```python
from build123d import *

# Parameters (mm, degrees)
SKETCH1_R           = 13.1
BOSS_EXTRUDE1_DEPTH = 47.8
SKETCH2_R           = 10
BOSS_EXTRUDE2_DEPTH = 0.4
SKETCH3_R           = 4
BOSS_EXTRUDE3_DEPTH = 1.4
CHAMFER2_SIZE       = 1.4
CHAMFER3_SIZE       = 0.4
SKETCH4_R           = 9
BOSS_EXTRUDE4_DEPTH = 0.4
CHAMFER4_SIZE       = 0.4
WRAP1_START         = 40.976923077
WRAP1_DEPTH         = 4.31474359
WRAP1_START_2       = 42.849358974
WRAP1_2_DEPTH       = 0.569871795
WRAP1_START_3       = 2.116666667
WRAP1_3_DEPTH       = 0.651282051


# Read off the part's stored shape, not the designer's step: Wrap1
with BuildPart() as part:
    # Sketch1 → Boss-Extrude1 (new body)
    with BuildSketch(Plane(origin=(0, 0, 0), x_dir=(1, 0, 0), z_dir=(0, 1, 0))):
        with Locations(Location((0, 0, 0), (0, 0, 90))):
            Circle(SKETCH1_R)
    extrude(amount=BOSS_EXTRUDE1_DEPTH)

    # Sketch2 → Boss-Extrude2 (add)
    with BuildSketch(Plane(origin=(0, 47.8, 0), x_dir=(1, 0, 0), z_dir=(0, 1, 0))):
        with Locations(Location((0, 0, 0), (0, 0, 270))):
            Circle(SKETCH2_R)
    extrude(amount=BOSS_EXTRUDE2_DEPTH)

    # Sketch3 → Boss-Extrude3 (add)
    with BuildSketch(Plane(origin=(0, 48.2, 0), x_dir=(1, 0, 0), z_dir=(0, 1, 0))):
        with Locations(Location((0, 0, 0), (0, 0, 270))):
            Circle(SKETCH3_R)
    extrude(amount=BOSS_EXTRUDE3_DEPTH)

    # Chamfer2
    chamfer2_edges = [part.edges().sort_by_distance(p)[0] for p in [
        (0, 48.2, -4),
    ]]
    chamfer(chamfer2_edges, length=CHAMFER2_SIZE - 0.0001)  # a hair under: the kernel refuses the full size

    # Chamfer3
    chamfer3_edges = [part.edges().sort_by_distance(p)[0] for p in [
        (0, 47.8, -10),
    ]]
    chamfer(chamfer3_edges, length=CHAMFER3_SIZE - 0.0001)  # a hair under: the kernel refuses the full size

    # Sketch4 → Boss-Extrude4 (add)
    with BuildSketch(Plane.XZ):
        with Locations(Location((0, 0, 0), (0, 0, 90))):
            Circle(SKETCH4_R)
    extrude(amount=BOSS_EXTRUDE4_DEPTH)

    # Chamfer4
    chamfer4_edges = [part.edges().sort_by_distance(p)[0] for p in [
        (0, 0, -9),
    ]]
    chamfer(chamfer4_edges, length=CHAMFER4_SIZE - 0.0001)  # a hair under: the kernel refuses the full size

    # Wrap1 outline → Wrap1 (add)
    with BuildSketch(Plane(origin=(0, 0, 0), x_dir=(1, 0, 0), z_dir=(0, 1, 0)).offset(WRAP1_START)):
        with BuildLine():
            Line((2.348137979, -12.887833333), (2.34993045, -12.897671375))
            ThreePointArc((2.34993045, -12.897671375), (2.62988756, -12.843511647), (2.908600522, -12.783275911))
            Line((2.908600522, -12.783275911), (2.906381909, -12.773525128))
            ThreePointArc((2.906381909, -12.773525128), (2.627881543, -12.833714918), (2.348137979, -12.887833333))
        make_face()
    extrude(amount=WRAP1_DEPTH)

    # Wrap1 2 outline → Wrap1 2 (add)
    with BuildSketch(Plane(origin=(0, 0, 0), x_dir=(1, 0, 0), z_dir=(0, 1, 0)).offset(WRAP1_START_2)):
        with BuildLine():
            ThreePointArc((0.488721144, -13.100887437), (1.422958155, -13.032547337), (2.34993045, -12.897671375))
            Line((2.34993045, -12.897671375), (2.348137979, -12.887833333))
            ThreePointArc((2.348137979, -12.887833333), (1.421872756, -13.022606416), (0.488348359, -13.090894388))
            Line((0.488348359, -13.090894388), (0.488721144, -13.100887437))
        make_face()
        with BuildLine():
            Line((2.906381909, -12.773525128), (2.908600522, -12.783275911))
            ThreePointArc((2.908600522, -12.783275911), (3.813980922, -12.542952186), (4.699889571, -12.238592158))
            Line((4.699889571, -12.238592158), (4.696304606, -12.229256848))
            ThreePointArc((4.696304606, -12.229256848), (3.811071706, -12.533384716), (2.906381909, -12.773525128))
        make_face()
    extrude(amount=WRAP1_2_DEPTH)

    # Wrap1 3 outline → Wrap1 3 (add)
    with BuildSketch(Plane(origin=(0, 0, 0), x_dir=(1, 0, 0), z_dir=(0, 1, 0)).offset(WRAP1_START_3)):
        with BuildLine():
            ThreePointArc((0.488721144, -13.100887437), (1.584826216, -13.01385515), (2.669782951, -12.835277909))
            Line((2.669782951, -12.835277909), (2.667746504, -12.82548746))
            ThreePointArc((2.667746504, -12.82548746), (1.462330473, -13.018125425), (0.244216621, -13.097723399))
            Line((0.244216621, -13.097723399), (0.244403046, -13.107721661))
            ThreePointArc((0.244403046, -13.107721661), (0.366578022, -13.104873923), (0.488721144, -13.100887437))
        make_face()
    extrude(amount=WRAP1_3_DEPTH)


solid = part.part
```
Verification items for the finished model (mm, model axes). A direction names the side the tool comes from. Coordinates: 2 decimals unless noted, no trailing zeros. Loops run counter-clockwise (first coordinate to the right, second up) from the corner with the lowest first, then second, coordinate; pieces in that order, holes last. Notation, with made-up numbers: (-32.75, -12.5) - (-17.75, -12.5) arc R4 ccw to (-17.75, -6.5) - close; hole circle Ø8 at (-40, -31.5). An arc over 180 degrees is marked (long way). Answer as a JSON object with one key per item and string values.
(1) Access from +Z, -Z, +X, -X, +Y, -Y to the whole of each face (thin tool, end or side, straight path). Record for faces 1 (the flat face through (6, 0, -9)), 2 (the flat face through (0, -0.4, 0)), 3 (the flat face through (-4, 48.2, 4)).
Response:
{"face 1": "-Y", "face 2": "+Z, -Z, +X, -X, -Y", "face 3": "+Y"}
(2) Go/stop test with flat-tipped pins: pin 1 Ø1 at (x, z) = (-4, 9) entering from +Y; pin 2 Ø8 at (x, z) = (2.5, 9) entering from -Y; pin 3 Ø8 at (x, y) = (3, 25) entering from +Z; pin 4 Ø2 at (x, y) = (8, 41) entering from +Z. Record where each tip stops, or that it passes through.
Response:
{"pin 1": "stops at y = 48.2", "pin 2": "stops at y = -0.4", "pin 3": "stops at z = 13.1", "pin 4": "stops at z = 11.07"}
(3) Scan lines: line 1 along Y through (x, z) = (6, 5.5); line 2 along Z through (x, y) = (-0.25, 22.5); line 3 along Y through (x, z) = (-10, 3.5). Record each from-to range of solid material in increasing order.
Response:
{"line 1": "y = -0.4 to 48.2", "line 2": "z = -13.1 to 13.1", "line 3": "y = 0 to 47.8"}
(4) Cross-section at C-C, the plane y = 23.5. Record the boundary of the cut face in (x, z), then the cut area to 3 significant figures.
Response:
{"outline": "circle Ø26.2 at (0, 0)", "area": "539 mm²"}
